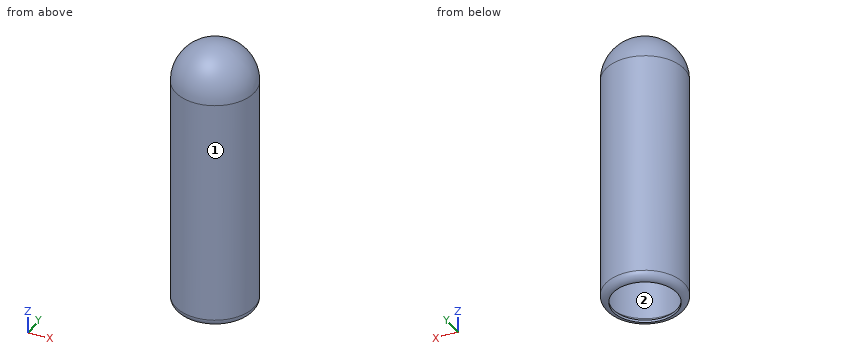
```python
from build123d import *

# Parameters (mm, degrees)
F2_T = -1.016


# Not quite as in the source:
# - a shell that OpenCascade refuses in one call is made with other operations: the cavity is built on its own and cut out


with BuildPart() as f1:
    # F0 (on Front) → F1 (revolve)
    with BuildSketch(Plane.XZ):
        with BuildLine():
            Line((0, 109.22), (0, 0))
            Line((0, 0), (12.7, 0))
            ThreePointArc((12.7, 0), (14.8013799323, 0.8704200677), (15.6718, 2.9718))
            Line((15.6718, 2.9718), (15.6718, 93.5482))
            ThreePointArc((15.6718, 93.5482), (11.0816360534, 104.6298360534), (0, 109.22))
        make_face()
    revolve(axis=Axis((0, 0, 54.61), (0, 0, 1)))

    # F2: a shell. OpenCascade refuses it in one call, so the cavity is built on its own and cut out:
    # the body offset inwards by the wall thickness, plus a prism from it out through each open face.
    f2_core = offset(f1.part, amount=F2_T, mode=Mode.PRIVATE)
    f2_exits = [f2_core.faces().sort_by_distance(p)[0] for p in [
        (0, 0, 1.016),
    ]]
    add(f2_core, mode=Mode.SUBTRACT)
    extrude(f2_exits, amount=-F2_T, mode=Mode.SUBTRACT)


solid = f1.part
```
Design review of the part built by this model. Coordinates are the model's own, in mm. Face numbers are marked on the shaded views. Coordinates: 2 decimals unless noted, no trailing zeros. Order: outer loops, then holes, each group sorted by start corner. A loop starts at its lowest first (then second) coordinate and runs counter-clockwise, first axis right, second up. Notation, with made-up numbers: M -34.75,57 L 20.25,57 A12 cw 20.25,79 Z; hole C 31.5,-19 d6. An arc over 180 degrees is marked long. Answer as a JSON object with one key per item and string values. Group by question number.
1) Add section C-C, the plane z = 89. Write out the cut boundary in (x, y).
2) Wall thickness on L1, parallel to Y at x = 0, z = 26; L2, parallel to Y at x = -0.5, z = 80: over which ranges is each line inside the solid? List them lowest first.
3) Add section A-A, the plane y = 0. Write out the cut boundary in (x, z).
4) Mouldability with a two-part tool opening along Z and no side actions: class the marked faces 1 and 2 as pulls with the +Z half, pulls with the -Z half, needs draft (parallel to the pull), parting line crosses it, or undercut.
5) For pin 1 (2 mm diameter, centred on x = -5.5, y = -6, fed in from -Z); pin 2 (1.5 mm diameter, centred on x = -4.5, z = 59, fed in from +Y); pin 3 (2 mm diameter, centred on x = -7, y = -5, fed in from +Z); pin 4 (6 mm diameter, centred on x = 10, y = -12, fed in from -Z), all flat-tipped, find the tip position at first contact; note any pin that passes through.
Computed values:
{
 "1": {"outline": "C 0,0 d31.34; hole C 0,0 d29.31"},
 "2": {"L1": "y = -15.67 to -14.66, 14.66 to 15.67", "L2": "y = -15.66 to -14.65, 14.65 to 15.66"},
 "3": {"outline": "M -15.67,2.97 A2.97 ccw -12.7,0 L -12.7,1.02 A1.96 cw -14.66,2.97 L -14.66,93.55 A14.66 cw 14.66,93.55 L 14.66,2.97 A1.96 cw 12.7,1.02 L 12.7,0 A2.97 ccw 15.67,2.97 L 15.67,93.55 A15.67 ccw -15.67,93.55 Z"},
 "4": {"face 1": "needs draft", "face 2": "undercut"},
 "5": {"pin 1": "stops at z = 105.01", "pin 2": "stops at y = 15.22", "pin 3": "stops at z = 107.25", "pin 4": "stops at z = 0"}
}
